The model under review builds one solid part; all positions refer to its coordinate system, in mm. A direction names the side the tool comes from. Round coordinates to 2 decimals unless told otherwise and drop trailing zeros. Order: outer loops, then holes, each group sorted by start corner. A loop starts at its lowest first (then second) coordinate and runs counter-clockwise, first axis right, second up. Notation, with made-up numbers: (-22, -27.75) -> (17, -27.75) arc R32 ccw to (17, 4.25) -> close; hole circle Ø8 at (71.5, -34). An arc over 180 degrees is marked (long way). Use a Markdown table: item, result. Add a question column.
```python
from build123d import *

# Parameters (mm, degrees)
SKETCH001_R          = 1.524
POCKET_DEPTH         = 4.064
SKETCH002_R          = 0.7874
POCKET001_DEPTH      = 15.073
SKETCH003_W          = 2.286
SKETCH003_H          = 5.08
POCKET002_DEPTH      = 5.0038
POCKET002_DEPTH_BACK = -99.9998


with BuildPart() as part:
    # Sketch → Revolution (revolve)
    with BuildSketch(Plane.XZ):
        Polygon((2.5, 0), (4, 0), (4, -4.572), (0, -4.572), (0, 0), (0, 10.5), (1.9, 10.5), (1.4, 9.15), (2.6, 3.5), (2.5, 2.5), align=None)
    revolve(axis=Axis((0, 0, 0), (0, 0, 1)))

    # Sketch001 (on Face5 of Revolution) → Pocket (cut)
    with BuildSketch(Plane(origin=(0, 0, -4.572), x_dir=(1, 0, 0), z_dir=(0, 0, -1))):
        Circle(SKETCH001_R)
    extrude(amount=-POCKET_DEPTH, mode=Mode.SUBTRACT)

    # Sketch002 (on Face6 of Pocket) → Pocket001 (cut, through all)
    with BuildSketch(Plane(origin=(0, 0, 10.5), x_dir=(-1, 0, 0), z_dir=(0, 0, 1))):
        Circle(SKETCH002_R)
    extrude(amount=-POCKET001_DEPTH, mode=Mode.SUBTRACT)

    # Sketch003 → Pocket002 (cut, two sides)
    with BuildSketch(Plane.XZ) as pocket002_sk:
        with Locations((0, -4.064)):
            Rectangle(SKETCH003_W, SKETCH003_H)
    extrude(amount=-POCKET002_DEPTH, mode=Mode.SUBTRACT)
    extrude(pocket002_sk.sketch, amount=-POCKET002_DEPTH_BACK, mode=Mode.SUBTRACT)


solid = part.part
```
Q1. Add section C-C (x = 0). Write out the cut boundary in (y, z).
Q2. Mouldability with a two-part tool opening along X and no side actions: class faces 1 (the flat face through (0.7, 0.7, -0.508)), 2 (the flat face through (-2, 2, 0)), 3 (the cylindrical face through (3.695, -1.532, -2.318)) as pulls with the +X half, pulls with the -X half, needs draft (parallel to the pull), parting line crosses it, or undercut.
Q3. Wall thickness on line 1 (Z direction, x = -2.5, y = 2.5); line 2 (X direction, y = 0, z = 3.75); line 3 (Z direction, x = -0.5, y = 2.75): over which ranges is each line inside the solid? List them lowest first. Write a range as [from, to].
Q4. Add section B-B (z = -3). Write out the cut boundary in (x, y), then the cut area to 3 significant figures.
Q5. Machinability: for faces 4 (the cylindrical face through (1.4, 0.6, -2.1)), 5 (the conical face through (-0.329, 2.506, 2.771)), 6 (the flat face through (0, 3, -1.524)), 7 (the cylindrical face through (0.625, 0.479, 5.073)), 8 (the flat face through (2, 0, -4.572)), which of the approach directions +Z, -Z, +X, -X, +Y, -Y give a long, thin tool a straight path to every point of the face, cutting with its end or side? Answer none if there is none.
Q6. Add section D-D (z = -1). Write out the cut boundary in (x, y), then the cut area to 3 significant figures.
Q7. Add section A-A (y = 0). Write out the cut boundary in (x, z).
Q8. Insertion check: pin 1 (4 mm diameter, centred on x = 1.5, z = 7.5, fed in from -Y); pin 2 (1.1 mm diameter, centred on x = 0, y = 2.5, fed in from -Z); pin 3 (1.4 mm diameter, centred on y = 3, z = -2.5, fed in from -X). Each pin has a flat end and moves straight along its axis. Give the tip position at first contact, or say it passes through.
Report:
| question | item | result |
|---|---|---|
| 1 | outline | (-4, -1.52) -> (-1.52, -1.52) -> (-1.52, -0.51) -> (-0.79, -0.51) -> (-0.79, 10.5) -> (-1.9, 10.5) -> (-1.4, 9.15) -> (-2.6, 3.5) -> (-2.5, 2.5) -> (-2.5, 0) -> (-4, 0) -> close; (0.79, -0.51) -> (1.52, -0.51) -> (1.52, -1.52) -> (4, -1.52) -> (4, 0) -> (2.5, 0) -> (2.5, 2.5) -> (2.6, 3.5) -> (1.4, 9.15) -> (1.9, 10.5) -> (0.79, 10.5) -> close |
| 2 | face 1 | undercut |
| 2 | face 2 | needs draft |
| 2 | face 3 | parting line crosses it |
| 3 | line 1 | z = [-4.57, 0] |
| 3 | line 2 | x = [-2.55, -0.79], [0.79, 2.55] |
| 3 | line 3 | z = [-1.52, 0] |
| 4 | outline | (-1.14, -3.83) -> (-1.14, -1.01) arc R1.52 cw to (-1.14, 1.01) -> (-1.14, 3.83) arc R4 ccw to start; (1.14, -3.83) arc R4 ccw to (1.14, 3.83) -> (1.14, 1.01) arc R1.52 cw to (1.14, -1.01) -> close |
| 4 | area | 31.2 mm² |
| 5 | face 4 | -Z |
| 5 | face 5 | none |
| 5 | face 6 | -Z, +Y, -Y |
| 5 | face 7 | +Z, -Z |
| 5 | face 8 | -Z, +X, -X, +Y, -Y |
| 6 | outline | circle Ø8 at (0, 0); hole circle Ø3.05 at (0, 0) |
| 6 | area | 43.0 mm² |
| 7 | outline | (-4, -4.57) -> (-1.52, -4.57) -> (-1.52, -0.51) -> (-0.79, -0.51) -> (-0.79, 10.5) -> (-1.9, 10.5) -> (-1.4, 9.15) -> (-2.6, 3.5) -> (-2.5, 2.5) -> (-2.5, 0) -> (-4, 0) -> close; (0.79, -0.51) -> (1.52, -0.51) -> (1.52, -4.57) -> (4, -4.57) -> (4, 0) -> (2.5, 0) -> (2.5, 2.5) -> (2.6, 3.5) -> (1.4, 9.15) -> (1.9, 10.5) -> (0.79, 10.5) -> close |
| 8 | pin 1 | stops at y = -2.07 |
| 8 | pin 2 | stops at z = -1.52 |
| 8 | pin 3 | stops at x = -3.27 |
